Could you check a few things on this model? Use its own coordinates, in mm. Give positions to 0.01 mm unless a question says otherwise; leave off trailing zeros. Order: outer loops, then holes, each group sorted by start corner. A loop starts at its lowest first (then second) coordinate and runs counter-clockwise, first axis right, second up. Notation, with made-up numbers: (51, -4) -> (98, -4) arc R14 ccw to (98, 16) -> close; hole circle Ø3 at (39, 44). An arc over 180 degrees is marked (long way). One line per item, written item: value.
```python
from build123d import *
from build123d.topology import SkipClean

# Parameters (mm, degrees)
BOSS_EXTRUDE1_DEPTH = 640
SKETCH22_R          = 6
CUT_EXTRUDE4_DEPTH  = 10
BOSS_EXTRUDE2_DEPTH = 63
BOSS_EXTRUDE3_DEPTH = 7
SKETCH26_R          = 6
CUT_EXTRUDE5_DEPTH  = 7


with BuildPart() as part:
    # Sketch1 → Boss-Extrude1 (new body)
    with BuildSketch(Plane.XY):
        Polygon((0, 0), (0, 70), (70, 70), (70, 63), (7, 63), (7, 0), align=None)
    extrude(amount=BOSS_EXTRUDE1_DEPTH)

    # Sketch22 → Cut-Extrude4 (cut)
    with BuildSketch(Plane(origin=(0, 70, 0), x_dir=(1, 0, 0), z_dir=(0, 1, 0))):
        with Locations((35, 0)):
            Circle(SKETCH22_R)
        with Locations((35, 500)):
            Circle(SKETCH22_R)
        with Locations(Location((35, -500, 0), (0, 0, 270))):
            Circle(SKETCH22_R)
    extrude(amount=-CUT_EXTRUDE4_DEPTH, mode=Mode.SUBTRACT)

    # Sketch23 → Boss-Extrude2 (add)
    with BuildSketch(Plane(origin=(0, 0, 0), x_dir=(1, 0, 0), z_dir=(0, 1, 0))):
        Polygon((0, -640), (42.5, -713.612159322), (48.562177826, -710.112159322), (7, -640), align=None)
    extrude(amount=BOSS_EXTRUDE2_DEPTH)

    # Sketch25 → Boss-Extrude3 (add)
    with BuildSketch(Plane(origin=(0, 63, 0), x_dir=(1, 0, 0), z_dir=(0, 1, 0))):
        Polygon((70, -640), (0, -640), (42.5, -713.612159322), (70, -713.612159322), align=None)
    extrude(amount=BOSS_EXTRUDE3_DEPTH)

    # Sketch26 → Cut-Extrude5 (cut)
    with BuildSketch(Plane(origin=(-275.556719825, 0, 163.348804279), x_dir=(-0.5099316128113042, 0, -0.8602149442178172), z_dir=(0.8602149442178172, 0, -0.5099316128113042))):
        with Locations((-614.36248118, 31.5)):
            Circle(SKETCH26_R)
        with Locations((-575.357085589, 31.5)):
            Circle(SKETCH26_R)
    extrude(amount=-CUT_EXTRUDE5_DEPTH, mode=Mode.SUBTRACT)

    # Mirror1: part across plane


with BuildPart() as part_1:
    with SkipClean():  # the faces are left unmerged after this step: merging them gives an invalid solid
        add(part.part)
        add(part.part.mirror(Plane.XY))


solid = part_1.part
```
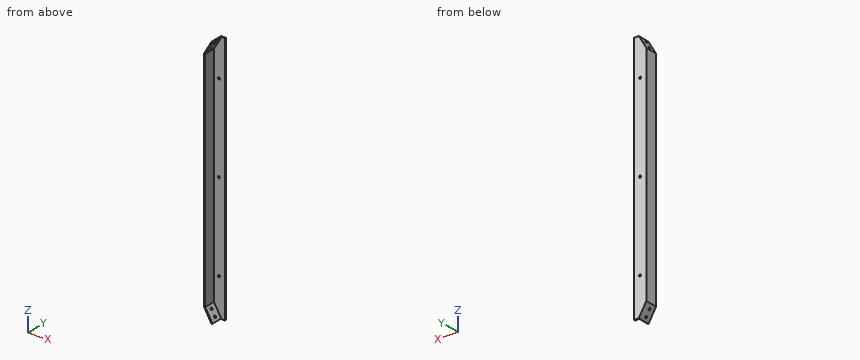
1) Suppose I cut it at A-A, the plane z = 528.5. Write out the boundary of the cut face in (x, y).
Answer below:
outline: (0, 0) -> (7, 0) -> (7, 63) -> (70, 63) -> (70, 70) -> (0, 70) -> close
2) If I drill on line 1 along X through (y, z) = (68, 500); line 2 along X through (y, z) = (8.5, 297.5); line 3 along Y through (x, z) = (42.5, -128.5), over which ranges is the centre line in solid material (lowest first)?
Answer below:
line 1: x = 0 to 29, 41 to 70
line 2: x = 0 to 7
line 3: y = 63 to 70
3) For P1, Ø10, axis at x = 19, y = 19, coming from the -Z side; P2, Ø3, axis at y = 29, z = -490.5, coming from the +X side; P3, Ø4, axis at x = 38.5, y = 19.5, coming from the +Z side; P4, Ø11, axis at x = 35, z = 0, coming from the -Y side, each with a flat end and sliding along its axis, tell me the tip position at first contact or that it passes through.
Answer below:
P1: stops at z = -681.57
P2: stops at x = 7
P3: stops at z = 710.15
P4: passes through
